Can you work these out from the drawing? Everything is in mm from the part's minimum corner. Round coordinates to 2 decimals unless told otherwise and drop trailing zeros. Loops run counter-clockwise (first coordinate to the right, second up) from the corner with the lowest first, then second, coordinate; pieces in that order, holes last. Notation, with made-up numbers: M 27,-32 L 71,-32 A20 cw 71,-6 Z; hole C 59,76 d1. An arc over 180 degrees is marked long. Return JSON: item names as keys, results as strings. Group by question number.
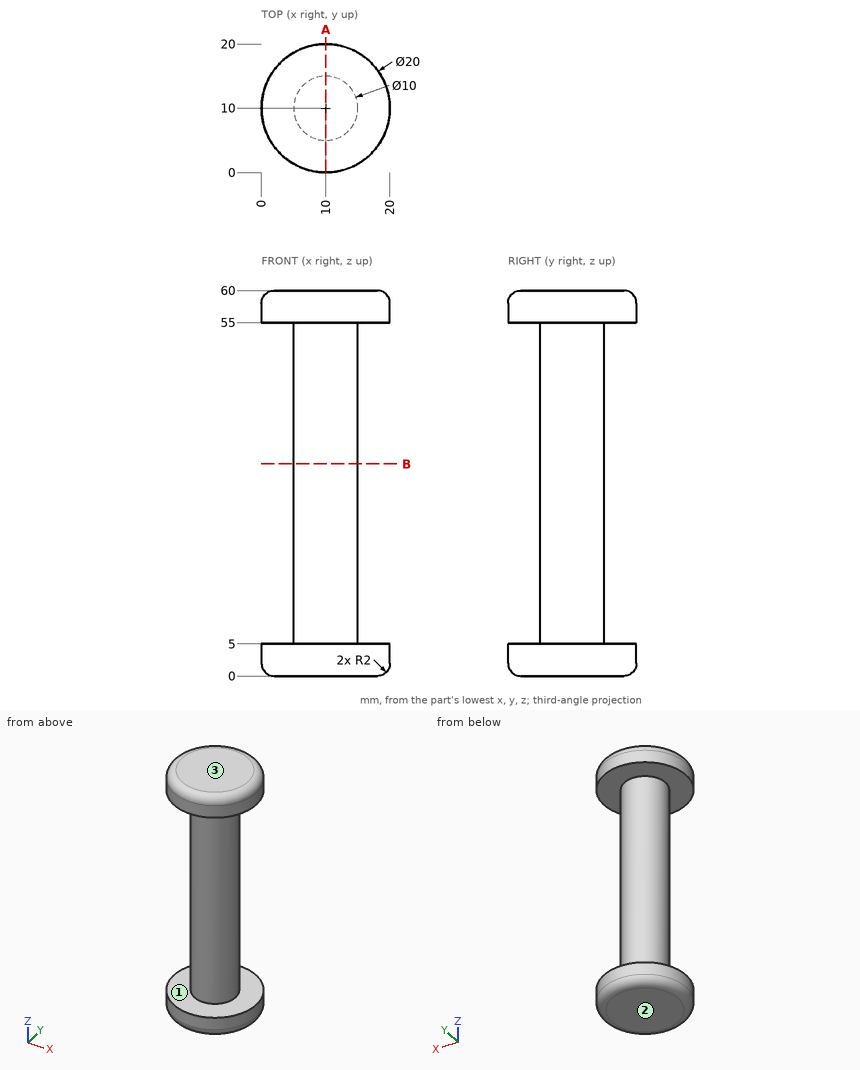
1. We'd pull the mould along Z, two halves only. Please class the marked faces 1, 2 and 3: +Z half, -Z half, draft (parallel to the pull), parting line (faces both ways), or undercut.
2. If we section it at A-A, the plane x = 10: Please give me the cut outline in (y, z), then the cut area to 3 significant figures.
3. I need wall thicknesses on probe 1 along Z at (x, y) = (15, 12.25); probe 2 along Z at (x, y) = (5.75, 18); probe 3 along Y at (x, z) = (13, 41). Which ranges of each line are inside material? Lowest first, please.
4. If we section it at B-B, the plane z = 33: Please give me the cut outline in (x, y).
5. I'm going to push flat-ended pins straight in: pin 1 Ø12 at (x, z) = (15, 44.5) entering from +Y; pin 2 Ø10 at (x, z) = (12.5, 54) entering from +Y; pin 3 Ø5 at (x, z) = (7.5, 38) entering from -Y; pin 4 Ø8 at (x, z) = (18, 23.5) entering from +Y. Where does each tip first touch, or does it pass through?
Geometry results:
{
 "1": {"face 1": "undercut", "face 2": "-Z half", "face 3": "+Z half"},
 "2": {"outline": "M 0,2 A2 ccw 2,0 L 18,0 A2 ccw 20,2 L 20,5 L 15,5 L 15,55 L 20,55 L 20,58 A2 ccw 18,60 L 2,60 A2 ccw 0,58 L 0,55 L 5,55 L 5,5 L 0,5 Z", "area": "697 mm^2"},
 "3": {"probe 1": "0 to 5, 55 to 60", "probe 2": "0.3 to 5, 55 to 59.7", "probe 3": "6 to 14"},
 "4": {"outline": "C 10,10 d10"},
 "5": {"pin 1": "y = 15", "pin 2": "y = 20", "pin 3": "y = 5", "pin 4": "y = 13"}
}
